```python
from build123d import *

# Parameters (mm, degrees)
F1_DEPTH = 20
F2_SIZE  = 19.99999
F3_SIZE  = 19.99999


# Not quite as in the source:
# - a fillet or chamfer is up to 0.001 mm smaller than in the source, because OpenCascade refuses the exact size


with BuildPart() as f1:
    # F0 (on Front) → F1 (new body)
    with BuildSketch(Plane.XZ):
        Polygon((-106.2891499103, -110.869043763), (71.5108500897, -110.869043763), (109.6108500897, 94.9895840839), (-144.3891499103, 94.9895840839), align=None)
    extrude(amount=F1_DEPTH)

    # F2 (size 20 in the source; OpenCascade refuses exactly that, so slightly less here)
    f2_edges = [f1.edges().sort_by_distance(p)[0] for p in [
        (90.56085, 0, -7.93973),
    ]]
    chamfer(f2_edges, length=F2_SIZE)

    # F3 (size 20 in the source; OpenCascade refuses exactly that, so slightly less here)
    f3_edges = [f1.edges().sort_by_distance(p)[0] for p in [
        (-125.33915, 0, -7.93973),
    ]]
    chamfer(f3_edges, length=F3_SIZE)


solid = f1.part
```
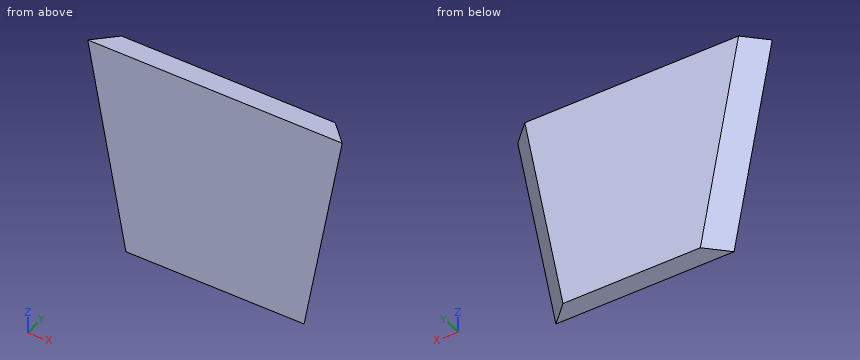
Geometry: final body of the model. Coordinates: model frame, mm. Round coordinates to 2 decimals unless told otherwise and drop trailing zeros. Write each loop counter-clockwise with the first axis right and the second up, starting at its lowest first coordinate (ties: lowest second). Pieces come first, ordered by that corner, then holes. Notation, with made-up numbers: (33.5, 50) -> (76.5, 50) arc R21 cw to (76.5, 71) -> close; hole circle Ø7 at (44.25, 51.5). An arc over 180 degrees is marked (long way). Return JSON: item names as keys, results as strings.
Q1. Section B-B on x = 62.5. Return the cut outline in (y, z), and give its area (3 significant figures).
From the geometry:
{"outline": "(-20, -110.87) -> (-11.14, -110.87) -> (0, -49.66) -> (0, 94.99) -> (-20, 94.99) -> close", "area": "3,780 mm2"}
Q2. Section C-C on y = -5.5. Return the cut outline in (x, z), and give its area (3 significant figures).
From the geometry:
{"outline": "(-129.64, 94.99) -> (-91.54, -110.87) -> (56.76, -110.87) -> (94.86, 94.99) -> close", "area": "38,400 mm2"}
Q3. First-contact query: pin 1 Ø1.5 at (y, z) = (-6.5, 54) entering from -X; pin 2 Ø8 at (y, z) = (-14, -36) entering from +X. Flat tips, straight axial feed; report the tip coordinate or a pass-through.
From the geometry:
{"pin 1": "x = -123.85", "pin 2": "x = 83.4"}
Q4. Ray query, line 1 (X direction, y = -13.75, z = 19.5); line 2 (X direction, y = -5.5, z = -9). Return the intervals inside material, ascending.
From the geometry:
{"line 1": "-124.06 to 89.28", "line 2": "-110.4 to 75.62"}
